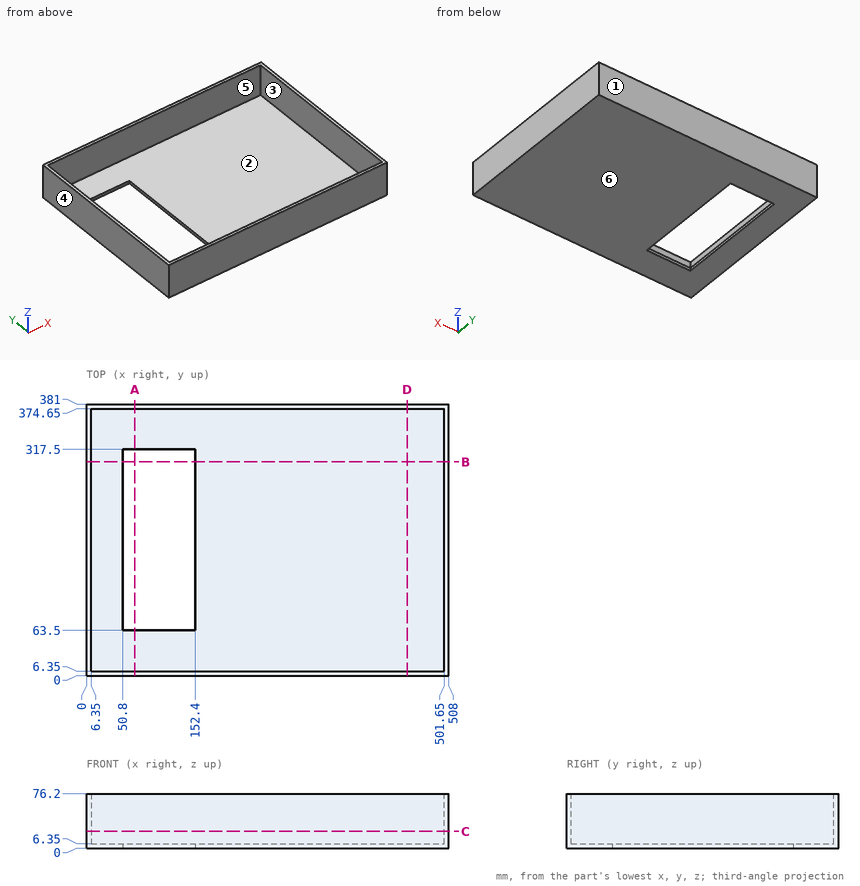
Geometry check sheet. Reference: drawing and pictorial views, mm from the part's lowest x, y, z. A direction names the side the tool comes from. Round coordinates to 2 decimals unless told otherwise and drop trailing zeros. Loops run counter-clockwise (first coordinate to the right, second up) from the corner with the lowest first, then second, coordinate; pieces in that order, holes last. Notation, with made-up numbers: (85, 6) - (104, 6) arc R11 cw to (104, 15) - close; hole circle Ø4 at (24, 49). An arc over 180 degrees is marked (long way). Use a Markdown table: item, result. Add a question column.
1. Section check D-D, the plane x = 449.5. Record the boundary of the cut face in (y, z).
2. Gauge pin test, flat end, axial feed: pin 1 (3 mm diameter, centred on x = 335.5, y = 267.5, fed in from +Z). Record the tip position at first contact, or that the pin passes through.
3. Section check C-C, the plane z = 23.5. Record the boundary of the cut face in (x, y), plus the area to 3 significant figures.
4. Section check B-B, the plane y = 300. Record the boundary of the cut face in (x, z).
5. Thickness scan on probe 1 along Y at (x, z) = (410, 50); probe 2 along X at (y, z) = (27.5, 38); probe 3 along X at (y, z) = (127.5, 5). Record the ranges inside material, lowest first. Write a range as [from, to].
6. Release check for a two-part mould opening along Y. For the marked faces 1, 2, 3 and 4 record: released by +Y, released by -Y, zero draft, split by the parting line, or undercut.
7. Access from +Z, -Z, +X, -X, +Y, -Y to the whole of each face (thin tool, end or side, straight path). Record for the marked faces 5 and 6.
8. Section check A-A, the plane x = 68. Record the boundary of the cut face in (y, z).
Checks:
| question | item | result |
|---|---|---|
| 1 | outline | (0, 0) - (381, 0) - (381, 76.2) - (374.65, 76.2) - (374.65, 6.35) - (6.35, 6.35) - (6.35, 76.2) - (0, 76.2) - close |
| 2 | pin 1 | stops at z = 6.35 |
| 3 | outline | (0, 0) - (508, 0) - (508, 381) - (0, 381) - close; hole (6.35, 6.35) - (501.65, 6.35) - (501.65, 374.65) - (6.35, 374.65) - close |
| 3 | area | 11,100 mm^2 |
| 4 | outline | (0, 0) - (50.8, 0) - (50.8, 6.35) - (6.35, 6.35) - (6.35, 76.2) - (0, 76.2) - close; (152.4, 0) - (508, 0) - (508, 76.2) - (501.65, 76.2) - (501.65, 6.35) - (152.4, 6.35) - close |
| 5 | probe 1 | y = [0, 6.35], [374.65, 381] |
| 5 | probe 2 | x = [0, 6.35], [501.65, 508] |
| 5 | probe 3 | x = [0, 50.8], [152.4, 508] |
| 6 | face 1 | released by +Y |
| 6 | face 2 | undercut |
| 6 | face 3 | undercut |
| 6 | face 4 | zero draft |
| 7 | face 5 | +Z |
| 7 | face 6 | -Z, +X, -X, +Y, -Y |
| 8 | outline | (0, 0) - (63.5, 0) - (63.5, 6.35) - (6.35, 6.35) - (6.35, 76.2) - (0, 76.2) - close; (317.5, 0) - (381, 0) - (381, 76.2) - (374.65, 76.2) - (374.65, 6.35) - (317.5, 6.35) - close |
